The model under review builds one solid part; all positions refer to its coordinate system, in mm. A direction names the side the tool comes from. Round coordinates to 2 decimals unless told otherwise and drop trailing zeros. Order: outer loops, then holes, each group sorted by start corner. A loop starts at its lowest first (then second) coordinate and runs counter-clockwise, first axis right, second up. Notation, with made-up numbers: (46.25, 53) -> (69.25, 53) arc R11 cw to (69.25, 65) -> close; hole circle Ø2 at (9, -25). An arc over 180 degrees is marked (long way). Use a Markdown table: item, result. Add a question column.
```python
from build123d import *

# Parameters (mm, degrees)
SKETCH_1_R          = 10
SKETCH_1_R_2        = 3
SKETCH_1_R_3        = 1.5
EXTRUDE_1_DEPTH     = 2
SKETCH_2_R          = 3
EXTRUDE_2_DEPTH     = 10
SKETCH_5_R          = 1.5
CUT_EXTRUDE_3_DEPTH = 5


with BuildPart() as part:
    # Sketch 1 → Extrude 1 (new body)
    with BuildSketch(Plane(origin=(0, 0, 0), x_dir=(1, 0, 0), z_dir=(0, 1, 0))):
        with Locations(Location((0, 0, 0), (0, 0, 270))):
            Circle(SKETCH_1_R)
        with Locations(Location((0, 0, 0), (0, 0, 270))):
            Circle(SKETCH_1_R_2, mode=Mode.SUBTRACT)
        with Locations(Location((0, 7, 0), (0, 0, 270))):
            Circle(SKETCH_1_R_3, mode=Mode.SUBTRACT)
        with Locations(Location((7, 0, 0), (0, 0, 270))):
            Circle(SKETCH_1_R_3, mode=Mode.SUBTRACT)
        with Locations(Location((0, -7, 0), (0, 0, 270))):
            Circle(SKETCH_1_R_3, mode=Mode.SUBTRACT)
        with Locations(Location((-7, 0, 0), (0, 0, 270))):
            Circle(SKETCH_1_R_3, mode=Mode.SUBTRACT)
    extrude(amount=EXTRUDE_1_DEPTH)

    # Sketch 2 → Extrude 2 (add)
    with BuildSketch(Plane(origin=(0, 0, 0), x_dir=(1, 0, 0), z_dir=(0, 1, 0))):
        with Locations(Location((0, 0, 0), (0, 0, 270))):
            Circle(SKETCH_2_R)
    extrude(amount=EXTRUDE_2_DEPTH)

    # Sketch 5 → Cut-Extrude 3 (cut, symmetric)
    with BuildSketch(Plane(origin=(0, 0, 0), x_dir=(0, 1, 0), z_dir=(0.7071067811865438, 0, -0.7071067811865512))):
        with Locations(Location((6, 0, 0), (0, 0, 270))):
            Circle(SKETCH_5_R)
    extrude(amount=CUT_EXTRUDE_3_DEPTH, both=True, mode=Mode.SUBTRACT)


solid = part.part
```
Q1. Add section C-C (z = -7). Write out the cut boundary in (x, y).
Q2. Insertion check: pin 1 (1 mm diameter, centred on x = -0.5, y = 7, fed in from +Z); pin 2 (5 mm diameter, centred on y = 2.5, z = -4.5, fed in from -X); pin 3 (6 mm diameter, centred on x = 6.5, z = 5, fed in from +Y). Each pin has a flat end and moves straight along its axis. Give the tip position at first contact, or say it passes through.
Q3. Add section B-B (y = 1.25). Write out the cut boundary in (x, z), then the cut area to 3 significant figures.
Q4. Wall thickness on line 1 (Y direction, x = 5.25, z = 6.5); line 2 (X direction, y = 1.75, z = 6.5); line 3 (X direction, y = 1.65, z = 7): over which ranges is each line inside the solid? List them lowest first. Write a range as [from, to].
Q5. Machinability: for faces 5 (the flat face through (0, 10, 0)), 6 (the cylindrical face through (0, 6, -3)), which of the approach directions +Z, -Z, +X, -X, +Y, -Y give a long, thin tool a straight path to every point of the face, cutting with its end or side? Answer none if there is none.
Q6. Add section D-D (z = 0.5). State how many separate pieces and enclosed holes the cut face has, then the cut area to 3 significant figures.
Q7. Add section A-A (x = -6.75). Write out the cut boundary in (y, z), then the cut area to 3 significant figures.
Q8. Mouldability with a two-part tool opening along X and no side actions: class faces 1 (the cylindrical face through (-9.76, 0.99, -2.17)), 2 (the cylindrical face through (0.07, 0.99, 5.5)), 3 (the flat face through (-2.1, 2, -2.4)), 4 (the cylindrical face through (-8.464, 0.986, -0.325)) as pulls with the +X half, pulls with the -X half, needs draft (parallel to the pull), parting line crosses it, or undercut.
Report:
| question | item | result |
|---|---|---|
| 1 | outline | (-7.14, 0) -> (-1.5, 0) -> (-1.5, 2) -> (-7.14, 2) -> close; (1.5, 0) -> (7.14, 0) -> (7.14, 2) -> (1.5, 2) -> close |
| 2 | pin 1 | stops at z = 3 |
| 2 | pin 2 | stops at x = -9.79 |
| 2 | pin 3 | stops at y = 2 |
| 3 | outline | circle Ø20 at (0, 0); hole circle Ø3 at (-7, 0); hole circle Ø3 at (0, -7); hole circle Ø3 at (0, 7); hole circle Ø3 at (7, 0) |
| 3 | area | 286 mm² |
| 4 | line 1 | y = [0, 2] |
| 4 | line 2 | x = [-7.6, -1.41], [1.41, 7.6] |
| 4 | line 3 | x = [-7.14, -1.5], [1.5, 7.14] |
| 5 | face 5 | +Z, -Z, +X, -X, +Y |
| 5 | face 6 | +Y |
| 6 | separate pieces | 3 |
| 6 | enclosed holes | 1 |
| 6 | area | 66.0 mm² |
| 7 | outline | (0, -7.38) -> (2, -7.38) -> (2, -1.48) -> (0, -1.48) -> close; (0, 1.48) -> (2, 1.48) -> (2, 7.38) -> (0, 7.38) -> close |
| 7 | area | 23.6 mm² |
| 8 | face 1 | parting line crosses it |
| 8 | face 2 | undercut |
| 8 | face 3 | needs draft |
| 8 | face 4 | undercut |
